Can you work these out from the model? Positions are in its coordinate system, mm. A direction names the side the tool comes from. Round coordinates to 2 decimals unless told otherwise and drop trailing zeros. Write each loop counter-clockwise with the first axis right and the second up, starting at its lowest first coordinate (ties: lowest second). Pieces come first, ordered by that corner, then holes. Notation, with made-up numbers: (35.5, 82) -> (76.5, 82) arc R25 cw to (76.5, 106) -> close; hole circle Ø7 at (33.25, -35). An arc over 180 degrees is marked (long way). Write item = value, one per line. Start each with the question number.
1) For faces 4 (the face through (4.1, -3.2, 79.8)), 5 (the face through (-2.75, 12.4, -1.4)), which set-ups out of +Z, -Z, +X, -X, +Y, -Y let a thin tool reach every point of the face, with its end or its side?
2) Imagine slicing it at A-A, the plane z = 62. Please give me the cut outline in (x, y) (1 decimal), then the cut area to 3 significant figures.
3) I'm going to push flat-ended pins straight in: pin 1 (4 mm diameter, centred on x = -7, z = -2.5, fed in from +Y); pin 2 (2.5 mm diameter, centred on x = 0, y = 8, fed in from +Z); pin 3 (2.5 mm diameter, centred on x = -8, y = 0, fed in from -Z). Where does each tip first touch, or does it pass through?
4) If I drill on line 1 (Y direction, x = 0, z = -88.75); line 2 (Y direction, x = 0.5, z = -20.5); line 3 (Y direction, x = 1.25, z = 67.5), over which ranges is the centre line in solid material (lowest first)?
5) Thinking about a two-plate mould opening in Z: for faces 1 (the face through (5.5, 0.2, 100)), 2 (the face through (5.5, 0.2, -100)), 3 (the face through (4.1, 3.2, -79.8)), which applies, +Z half, -Z half, draft (parallel to the pull), parting line (faces both ways), or undercut?
Autodesk Inventor part; units mm, degrees
ref_plane "Work Plane1" through (0, 0, -80) normal (0, 0, -1) x (-1, 0, 0)
ref_plane "YZ Plane" through (0, 0, 0) normal (1, 0, 0) x (0, 1, 0)
ref_plane "XZ Plane" through (0, 0, 0) normal (0, 1, 0) x (-1, 0, 0)
sketch "Sketch1" plane through (0, 0, 0) normal (0, 0, 1) x (1, 0, 0)
  circle A0 centre (0, 0) radius 12.7
  circle A1 centre (0, 0) radius 5
  dimension "d0" = 25.4
  dimension "d1" = 10
extrude "Extrusion1" add sketch "Sketch1" along normal mid plane 200
sketch "Sketch2" plane through (0, 0, 100) normal (0, 0, 1) x (1, 0, 0)
  line L0 (-17.78, 0) -> (17.78, 0)
  line L1 (0, -17.78) -> (0, 17.78)
  circle A0 centre (0, 0) radius 8 construction
  line L2 (0, 0) -> (8, 0) construction
  circle A1 centre (0, 8) radius 1.5
  circle A2 centre (-8, 0) radius 1.5
  circle A3 centre (0, -8) radius 1.5
  circle A4 centre (8, 0) radius 1.5
  point P0 (8, 0)
  point P1 (0, -8)
  point P2 (-8, 0)
  dimension "d4" = 16
  dimension "d25" = 3
  dimension "d28" = 360
extrude "Extrusion3" cut sketch "Sketch2" against normal blind 15
thread "Thread1"
thread "Thread2"
thread "Thread3"
thread "Thread4"
mirror "Mirror2" about plane through (0, 0, 0) normal (0, 0, 1) of "Extrusion3"
thread "Thread5"
thread "Thread6"
thread "Thread7"
thread "Thread8"
ref_plane "Work Plane1" through (0, 0, -80) normal (0, 0, -1) x (-1, 0, 0)
sketch "Sketch3" plane through (0, 0, -80) normal (0, 0, -1) x (-1, 0, 0)
  circle A0 centre (0, 0) radius 7.9375
  dimension "d49" = 15.875
extrude "Extrusion4" cut sketch "Sketch3" against normal blind 160
chamfer "Chamfer3" distance 2.9375 angle 45 2 edges at (7.9375, 0, 80) (7.9375, 0, -80)
properties part number "barra solida hueca para imprimir 3D"
Reported:
q1.face_4 = none
q1.face_5 = +Z, -Z
q2.outline = circle Ø25.4 at (0, 0); hole circle Ø15.9 at (0, 0)
q2.area = 309 mm²
q3.pin_1 = 11.67
q3.pin_2 = 85
q3.pin_3 = -85
q4.line_1 = -12.7 to -9.5, -6.5 to -5, 5 to 6.5, 9.5 to 12.7
q4.line_2 = -12.69 to -7.92, 7.92 to 12.69
q4.line_3 = -12.64 to -7.84, 7.84 to 12.64
q5.face_1 = +Z half
q5.face_2 = -Z half
q5.face_3 = undercut
